```python
from build123d import *

# Parameters (mm, degrees)
SKETCH_1_W          = 55
SKETCH_1_H          = 65
EXTRUDE_1_DEPTH     = 5
SKETCH_2_W          = 3
SKETCH_2_H          = 15
CUT_EXTRUDE_1_DEPTH = 86.293610546
SKETCH_4_R          = 7.5
CUT_EXTRUDE_2_DEPTH = 86.293610546
SKETCH_5_R          = 1.5
SKETCH_5_R_2        = 1.6
CUT_EXTRUDE_3_DEPTH = 86.293610546
SKETCH_6_R          = 1
CUT_EXTRUDE_4_DEPTH = 86.293610546


with BuildPart() as part:
    # 草图1 → 凸台-拉伸1 (new body)
    with BuildSketch(Plane.XY):
        with Locations((27.5, 32.5)):
            Rectangle(SKETCH_1_W, SKETCH_1_H)
    extrude(amount=EXTRUDE_1_DEPTH)

    # 草图2 → 切除-拉伸1 (cut, through all)
    with BuildSketch(Plane.XY.offset(5)):
        with Locations((53.5, 47.5)):
            Rectangle(SKETCH_2_W, SKETCH_2_H)
        with Locations((53.5, 17.5)):
            Rectangle(SKETCH_2_W, SKETCH_2_H)
    extrude(amount=-CUT_EXTRUDE_1_DEPTH, mode=Mode.SUBTRACT)

    # 草图4 → 切除-拉伸2 (cut, through all)
    with BuildSketch(Plane.XY.offset(5)):
        with Locations((27.5, 32.5)):
            Circle(SKETCH_4_R)
    extrude(amount=-CUT_EXTRUDE_2_DEPTH, mode=Mode.SUBTRACT)

    # 草图5 → 切除-拉伸3 (cut, through all)
    with BuildSketch(Plane.XY.offset(5)):
        with Locations((3, 60)):
            Circle(SKETCH_5_R)
        with Locations((3, 10)):
            Circle(SKETCH_5_R_2)
    extrude(amount=-CUT_EXTRUDE_3_DEPTH, mode=Mode.SUBTRACT)

    # 草图6 → 切除-拉伸4 (cut, through all)
    with BuildSketch(Plane(origin=(0, 0, 0), x_dir=(-1, 0, 0), z_dir=(0, 0, -1))):
        with Locations((-53, 32.5)):
            Circle(SKETCH_6_R)
        with Locations((-53, 5)):
            Circle(SKETCH_6_R)
    extrude(amount=-CUT_EXTRUDE_4_DEPTH, mode=Mode.SUBTRACT)


solid = part.part
```
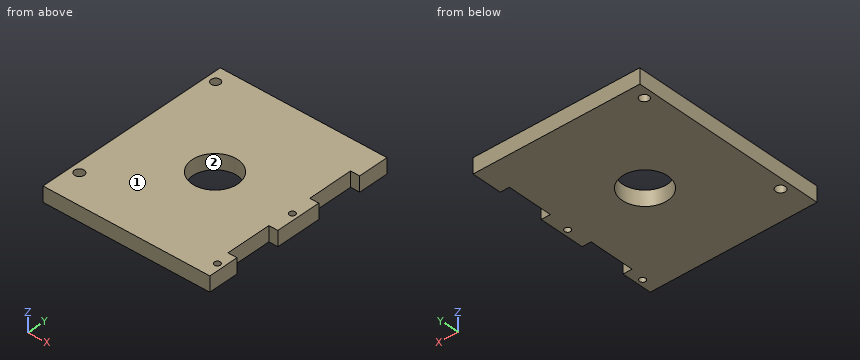
The model under review builds one solid part; all positions refer to its coordinate system, in mm. Face numbers are marked on the shaded views. Give positions to 0.01 mm unless a question says otherwise; leave off trailing zeros. Write each loop counter-clockwise with the first axis right and the second up, starting at its lowest first coordinate (ties: lowest second). Pieces come first, ordered by that corner, then holes. Notation, with made-up numbers: (-25.5, 53) - (11.5, 53) arc R34 ccw to (11.5, 89) - close; hole circle Ø4 at (63.5, 74.5). An arc over 180 degrees is marked (long way). Answer in a Markdown table with one row per item. Add a question column.
1. We need section A-A on y = 60. Write out the cut boundary in (x, z).
2. We need section C-C on z = 0.8. Write out the cut boundary in (x, y), then the cut area to 3 significant figures.
3. Wall thickness on line 1 along Y through (x, z) = (3, 3.85); line 2 along Y through (x, z) = (27.5, 1.95); line 3 along Y through (x, z) = (3.5, 2.45): over which ranges is each line inside the solid? List them lowest first. Write a range as [from, to].
4. We need section D-D on x = 27.5. Write out the cut boundary in (y, z), then the cut area to 3 significant figures.
5. Insertion check: P1, Ø2.5, axis at y = 45.5, z = 3.5, coming from the +X side; P2, Ø1.6, axis at x = 53, y = 5, coming from the +Z side. Each pin has a flat end and moves straight along its axis. Give the tip position at first contact, or say it passes through.
6. We need section B-B on x = 53. Write out the cut boundary in (y, z), then the cut area to 3 significant figures.
7. Draft analysis for pull direction Y (two halves, no side actions). For the marked faces 1 and 2, state which applies: +Y half, -Y half, draft (parallel to the pull), parting line (faces both ways), or undercut.
Ans:
| question | item | result |
|---|---|---|
| 1 | outline | (0, 0) - (1.5, 0) - (1.5, 5) - (0, 5) - close; (4.5, 0) - (55, 0) - (55, 5) - (4.5, 5) - close |
| 2 | outline | (0, 0) - (55, 0) - (55, 10) - (52, 10) - (52, 25) - (55, 25) - (55, 40) - (52, 40) - (52, 55) - (55, 55) - (55, 65) - (0, 65) - close; hole circle Ø3.2 at (3, 10); hole circle Ø3 at (3, 60); hole circle Ø15 at (27.5, 32.5); hole circle Ø2 at (53, 5); hole circle Ø2 at (53, 32.5) |
| 2 | area | 3,290 mm^2 |
| 3 | line 1 | y = [0, 8.4], [11.6, 58.5], [61.5, 65] |
| 3 | line 2 | y = [0, 25], [40, 65] |
| 3 | line 3 | y = [0, 8.48], [11.52, 58.59], [61.41, 65] |
| 4 | outline | (0, 0) - (25, 0) - (25, 5) - (0, 5) - close; (40, 0) - (65, 0) - (65, 5) - (40, 5) - close |
| 4 | area | 250 mm^2 |
| 5 | P1 | stops at x = 52 |
| 5 | P2 | passes through |
| 6 | outline | (0, 0) - (4, 0) - (4, 5) - (0, 5) - close; (6, 0) - (10, 0) - (10, 5) - (6, 5) - close; (25, 0) - (31.5, 0) - (31.5, 5) - (25, 5) - close; (33.5, 0) - (40, 0) - (40, 5) - (33.5, 5) - close; (55, 0) - (65, 0) - (65, 5) - (55, 5) - close |
| 6 | area | 155 mm^2 |
| 7 | face 1 | draft |
| 7 | face 2 | undercut |
